from build123d import *

# Parameters (mm, degrees)
F0_R     = 66.758219
F1_DEPTH = 101.6
F2_R     = 56.321266
F3_DEPTH = 101.6
F4_R     = 44.069911
F5_DEPTH = 82.55
F6_SIZE  = 5.08
F7_SIZE  = 2.54


with BuildPart() as f1:
    # F0 (on Front) → F1 (new body)
    with BuildSketch(Plane.XZ):
        Circle(F0_R)
    extrude(amount=F1_DEPTH)

    # F2 (on face) → F3 (join)
    with BuildSketch(Plane.XZ.offset(101.6)):
        Circle(F2_R)
    extrude(amount=F3_DEPTH)

    # F4 (on face) → F5 (join)
    with BuildSketch(Plane.XZ.offset(203.2)):
        Circle(F4_R)
    extrude(amount=F5_DEPTH)

    # F6
    f6_edges = [f1.edges().sort_by_distance(p)[0] for p in [
        (66.758219, -50.8, 0),
        (-66.758219, 0, 0),
        (-66.758219, -101.6, 0),
    ]]
    chamfer(f6_edges, length=F6_SIZE)

    # F7
    f7_edges = [f1.edges().sort_by_distance(p)[0] for p in [
        (56.321266, -152.4, 0),
        (-56.321266, -101.6, 0),
        (-56.321266, -203.2, 0),
        (44.069911, -244.475, 0),
        (-44.069911, -203.2, 0),
        (-44.069911, -285.75, 0),
    ]]
    chamfer(f7_edges, length=F7_SIZE)


solid = f1.part
Verification items for the finished model (mm, model axes). A direction names the side the tool comes from. Give positions to 0.01 mm unless a question says otherwise; leave off trailing zeros. Loops run counter-clockwise (first coordinate to the right, second up) from the corner with the lowest first, then second, coordinate; pieces in that order, holes last.
1) Sectioned sample at D-D, the plane y = -256. Enter the section's corners in (x, z), then the cut area to 3 significant figures.
2) Sectioned sample at C-C, the plane y = -125. Enter the section's corners in (x, z).
3) Sectioned sample at A-A, the plane x = 0. Enter the section's corners in (y, z).
4) Thickness scan on line 1 along Y through (x, z) = (51, 6.5); line 2 along X through (y, z) = (-208, -0.5); line 3 along Z through (x, y) = (25.5, -48). Record the ranges inside material, lowest first.
5) Set-up check for faces 1 (the cylindrical face through (-52.98, -50.16, -40.62)), 2 (the flat face through (-16, -203.2, 44)): record each of +Z, -Z, +X, -X, +Y, -Y from which the full face is reachable in a straight line by a thin tool's end or side.
6) Depth check by flat-ended pin: pin 1 Ø10 at (y, z) = (-204, 48.5) entering from -X; pin 2 Ø1 at (x, z) = (-39.5, -33.5) entering from -Y; pin 3 Ø12 at (y, z) = (-130, 51) entering from +X. Enter the tip coordinate at first touch or a pass-through.
7) Sectioned sample at B-B, the plane z = 0. Enter the section's corners in (x, y).
Answers:
1. outline: circle Ø88.14 at (0, 0)
1. area: 6,100 mm2
2. outline: circle Ø112.64 at (0, 0)
3. outline: (-285.75, -41.53) - (-283.21, -44.07) - (-205.74, -44.07) - (-203.2, -46.61) - (-203.2, -53.78) - (-200.66, -56.32) - (-104.14, -56.32) - (-101.6, -58.86) - (-101.6, -61.68) - (-96.52, -66.76) - (-5.08, -66.76) - (0, -61.68) - (0, 61.68) - (-5.08, 66.76) - (-96.52, 66.76) - (-101.6, 61.68) - (-101.6, 58.86) - (-104.14, 56.32) - (-200.66, 56.32) - (-203.2, 53.78) - (-203.2, 46.61) - (-205.74, 44.07) - (-283.21, 44.07) - (-285.75, 41.53) - close
4. line 1: y = -203.2 to 0
4. line 2: x = -44.07 to 44.07
4. line 3: z = -61.7 to 61.7
5. face 1: +Y, -Y
5. face 2: -Y
6. pin 1: stops at x = -34.16
6. pin 2: stops at y = -203.2
6. pin 3: stops at x = 33.87
7. outline: (-66.76, -96.52) - (-61.68, -101.6) - (-58.86, -101.6) - (-56.32, -104.14) - (-56.32, -200.66) - (-53.78, -203.2) - (-46.61, -203.2) - (-44.07, -205.74) - (-44.07, -283.21) - (-41.53, -285.75) - (41.53, -285.75) - (44.07, -283.21) - (44.07, -205.74) - (46.61, -203.2) - (53.78, -203.2) - (56.32, -200.66) - (56.32, -104.14) - (58.86, -101.6) - (61.68, -101.6) - (66.76, -96.52) - (66.76, -5.08) - (61.68, 0) - (-61.68, 0) - (-66.76, -5.08) - close
